Autodesk Inventor part; units mm, degrees
ref_plane "YZ Plane" through (0, 0, 0) normal (1, 0, 0) x (0, 1, 0)
ref_plane "XZ Plane" through (0, 0, 0) normal (0, 1, 0) x (-1, 0, 0)
ref_plane "XY Plane" through (0, 0, 0) normal (0, 0, 1) x (1, 0, 0)
sketch "Sketch1" plane through (0, 0, 0) normal (0, 0, 1) x (1, 0, 0)
  line L0 (-47.7435, -77.7913) -> (102.2565, -77.7913)
  line L1 (102.2565, -77.7913) -> (109.4965, -77.7913)
  line L2 (-47.7435, -77.7913) -> (-47.7435, -13.2313) construction
  line L3 (-47.7435, -13.2313) -> (-47.7435, 15.6487) construction
  line L4 (-47.7435, -77.7913) -> (-47.7435, -72.7913)
  line L5 (-47.7435, -72.7913) -> (-61.2235, -72.7913) construction
  line L6 (-47.7435, -72.7913) -> (-47.7435, -57.7913) construction
  line L7 (-47.7435, -57.7913) -> (-65.2735, -57.7913) construction
  line L8 (-47.7435, -57.7913) -> (-47.7435, -42.7913) construction
  line L9 (-47.7435, -42.7913) -> (-67.4235, -42.7913) construction
  line L10 (-47.7435, -42.7913) -> (-47.7435, -27.7913) construction
  line L11 (-47.7435, -27.7913) -> (-69.5835, -27.7913) construction
  line L12 (-47.7435, -27.7913) -> (-47.7435, -12.7913) construction
  line L13 (-47.7435, -12.7913) -> (-72.3735, -12.7913) construction
  line L14 (-47.7435, -77.7913) -> (42.2565, -77.7913)
  line L15 (42.2565, -77.7913) -> (42.2565, 92.2087) construction
  line L16 (42.2565, 92.2087) -> (-47.7435, 15.6487)
  line L17 (42.2565, 92.2087) -> (47.8065, 92.2087)
  line L18 (42.2565, -77.7913) -> (67.2565, -77.7913)
  line L19 (67.2565, -77.7913) -> (67.2565, -22.7913) construction
  line L20 (67.2565, -22.7913) -> (63.6956, -23.3847)
  line L21 (102.2565, -77.7913) -> (97.2565, -77.7913)
  line L22 (97.2565, -77.7913) -> (97.2565, -17.7913) construction
  line L23 (97.2565, -17.7913) -> (113.897, -15.0179)
  line L24 (109.4965, -77.7913) -> (113.897, -15.0179)
  line L25 (97.2565, -17.7913) -> (67.2565, -22.7913)
  line L26 (63.6956, -23.3847) -> (47.8065, 92.2087)
  spline S0 degree 2 poles (42.2565, 92.2087) (45.0586, 96.9623) (47.8065, 92.2087) knots 0 0 0 1 1 1
  line L27 (-59.7435, -93.9838) -> (-59.7435, 5.4407) construction
  line L28 (-47.7435, 15.6487) -> (-59.7435, 5.4407)
  line L29 (-59.7435, 5.4407) -> (-47.7435, -77.7913)
  line L30 (-69.5835, -27.7913) -> (-65.2735, -57.7913)
  line L31 (-47.7435, -77.7913) -> (-61.2235, -72.7913) construction
  line L32 (-61.2235, -72.7913) -> (-65.2735, -57.7913) construction
  spline S1 degree 2 poles (-47.7435, -77.7913) (-61.2235, -72.7913) (-65.2735, -57.7913) knots 1 1 1 2 2 2
  line L33 (-69.5835, -27.7913) -> (-72.3735, -12.7913) construction
  line L34 (-72.3735, -12.7913) -> (-59.7435, 5.4407) construction
  spline S2 degree 2 poles (-69.5835, -27.7913) (-72.3735, -12.7913) (-59.7435, 5.4407) knots 1 1 1 2 2 2
  line L35 (102.2565, -77.7913) -> (106.5714, -16.2388)
  line L36 (63.6956, -23.3847) -> (-52.7885, -42.7988)
  line L37 (-131.9637, -55.9946) -> (-133.7071, -56.2852)
  point P0 (0, 0)
  point P1 (45.0505, 94.5855)
  point P2 (-53.7435, 10.5447)
  dimension "d0" = 150
  dimension "d1" = 7.24
  dimension "d2" = 64.56
  dimension "d3" = 28.88
  dimension "d4" = 13.48
  dimension "d5" = 15
  dimension "d6" = 17.53
  dimension "d7" = 15
  dimension "d8" = 19.68
  dimension "d9" = 15
  dimension "d10" = 21.84
  dimension "d11" = 15
  dimension "d12" = 24.63
  dimension "d13" = 90
  dimension "d14" = 170
  dimension "d15" = 5.55
  dimension "d16" = 25
  dimension "d17" = 55
  dimension "d18" = 3.61
  dimension "d19" = 5
  dimension "d20" = 60
  dimension "d21" = 16.87
  dimension "d22" = 12
  dimension "d23" = 5
extrude "Extrusion1" add sketch "Sketch1" along normal mid plane 5.3 contours L29 L36 L20 L25 L23 L35 L0
extrude "Extrusion2" add sketch "Sketch1" along normal mid plane 5.4 contours L35 L23 L24 L1
chamfer "Chamfer1" distance 5 angle 20 1 edges at (26.8914, -29.5188, 2.65) measured on face at (52.0131, -45.6096, 2.65)
chamfer "Chamfer2" distance 5 angle 20 1 edges at (110.2342, -15.6283, 2.7) measured on face at (109.9883, -36.3493, 2.7)
chamfer "Chamfer3" distance 5 angle 20 1 edges at (26.8914, -29.5188, -2.65) measured on face at (52.0131, -45.6096, -2.65)
chamfer "Chamfer4" distance 5 angle 20 1 edges at (110.2342, -15.6283, -2.7) measured on face at (109.9883, -36.3493, -2.7)
fillet "Fillet1" radius 2 4 edges at (27.2565, -77.7913, -2.65) (105.8765, -77.7913, -2.7) (27.2565, -77.7913, 2.65) (105.8765, -77.7913, 2.7)
properties part number "vertical_stabilizer_01"
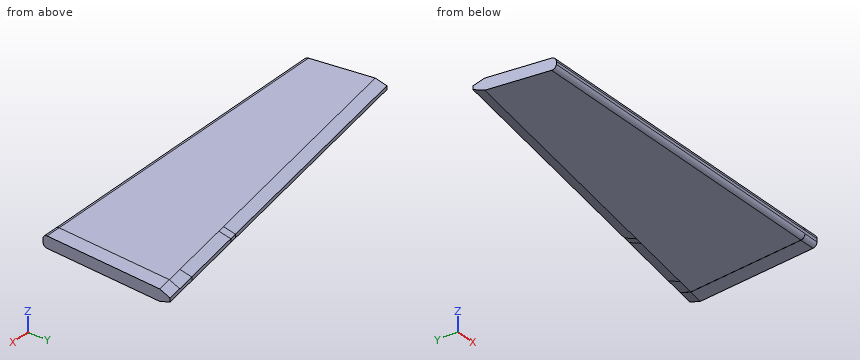
Geometry: final body of the model. Coordinates: model frame, mm. Coordinates: 2 decimals unless noted, no trailing zeros. Order: outer loops, then holes, each group sorted by start corner. A loop starts at its lowest first (then second) coordinate and runs counter-clockwise, first axis right, second up. Notation, with made-up numbers: (-15.75, 26.25) - (30.25, 26.25) arc R18 cw to (30.25, 57.25) - close; hole circle Ø9 at (-21.5, 23). An arc over 180 degrees is marked (long way). Use one line per item in the form item = value.
1) Ray query, L1, parallel to Z at x = -1, y = -39.5; L2, parallel to X at y = -57, z = -1.95; L3, parallel to Z at x = 15, y = -34. Return the intervals inside material, ascending.
Solutions:
L1 = -2.65 to 2.65
L2 = -50.74 to 110.95
L3 = -1.73 to 1.73
2) Section C-C (y = -32). Return loops of the section in (x, z), then the cut area to 3 significant figures.
Solutions:
outline = (12, -0.83) - (42.42, -2.65) - (105.47, -2.65) - (105.47, -2.7) - (112.71, -2.7) - (112.71, 2.7) - (105.47, 2.7) - (105.47, 2.65) - (42.42, 2.65) - (12, 0.83) - close
area = 479 mm^2
3) Section A-A (x = -29). Return loops of the section in (y, z).
Solutions:
outline = (-77.79, -0.65) arc R2 ccw to (-75.79, -2.65) - (-43.9, -2.65) - (-38.83, -0.83) - (-38.83, 0.83) - (-43.9, 2.65) - (-75.79, 2.65) arc R2 ccw to (-77.79, 0.65) - close
4) Section B-B (y = -70.5). Return loops of the section in (x, z).
Solutions:
outline = (-48.79, -2.65) - (102.77, -2.65) - (102.77, -2.7) - (110.01, -2.7) - (110.01, 2.7) - (102.77, 2.7) - (102.77, 2.65) - (-48.79, 2.65) - close
5) Pin query (flat end, axial travel): pin 1 (1 mm diameter, centred on x = 14.5, y = -61.5, fed in from -Z). Return the tip coordinate at first contact, or that it passes through.
Solutions:
pin_1 = -2.65
